Here's how the part is built. I have some questions about the finished solid (model axes, mm). A direction names the side the tool comes from. Give positions to 0.01 mm unless a question says otherwise; leave off trailing zeros. Loops run counter-clockwise (first coordinate to the right, second up) from the corner with the lowest first, then second, coordinate; pieces in that order, holes last. Notation, with made-up numbers: (-6.75, 2) - (44.25, 2) arc R19 cw to (44.25, 22) - close; hole circle Ø5 at (76, 9). An arc over 180 degrees is marked (long way). Use one line per item in the form item = value.
from build123d import *

# Parameters (mm, degrees)
SKETCH2_R           = 3.5
BOSS_EXTRUDE1_DEPTH = 8
SKETCH3_R           = 3.5
BOSS_EXTRUDE2_DEPTH = 18
SKETCH4_W           = 12.5
SKETCH4_H           = 8
SKETCH4_W_2         = 8.5
SKETCH4_H_2         = 4
BOSS_EXTRUDE3_DEPTH = 10
SKETCH5_W           = 12.5
SKETCH5_H           = 8
BOSS_EXTRUDE4_DEPTH = 1
FILLET2_R           = 2
SKETCH6_W           = 15.377134156
SKETCH6_H           = 9.300468084
CUT_EXTRUDE1_DEPTH  = 12


with BuildPart() as part:
    # Sketch2 → Boss-Extrude1 (new body)
    with BuildSketch(Plane.XY):
        Circle(SKETCH2_R)
        with BuildLine():
            Line((-1.237436867, -1.237436867), (1.237436867, -1.237436867))
            ThreePointArc((1.237436867, -1.237436867), (0, 1.75), (-1.237436867, -1.237436867))
        make_face(mode=Mode.SUBTRACT)
    extrude(amount=BOSS_EXTRUDE1_DEPTH)

    # Sketch3 → Boss-Extrude2 (add)
    with BuildSketch(Plane.XY.offset(8)):
        Circle(SKETCH3_R)
    extrude(amount=BOSS_EXTRUDE2_DEPTH)

    # Sketch4 → Boss-Extrude3 (add)
    with BuildSketch(Plane.XY.offset(26)):
        Rectangle(SKETCH4_W, SKETCH4_H)
        Rectangle(SKETCH4_W_2, SKETCH4_H_2, mode=Mode.SUBTRACT)
    extrude(amount=BOSS_EXTRUDE3_DEPTH)

    # Sketch5 → Boss-Extrude4 (add)
    with BuildSketch(Plane(origin=(0, 0, 26), x_dir=(-1, 0, 0), z_dir=(0, 0, -1))):
        Rectangle(SKETCH5_W, SKETCH5_H)
    extrude(amount=BOSS_EXTRUDE4_DEPTH)

    # Fillet2
    fillet2_edges = [part.edges().sort_by_distance(p)[0] for p in [
        (-6.25, -4, 30.5),
        (6.25, -4, 30.5),
        (6.25, 4, 30.5),
        (-6.25, 4, 30.5),
    ]]
    fillet(fillet2_edges, radius=FILLET2_R)

    # Sketch6 → Cut-Extrude1 (cut, through all)
    with BuildSketch(Plane(origin=(0, 0, 25), x_dir=(-1, 0, 0), z_dir=(0, 0, -1))):
        with Locations((-0.478823703, -0.270525698)):
            Rectangle(SKETCH6_W, SKETCH6_H)
    extrude(amount=-CUT_EXTRUDE1_DEPTH, mode=Mode.SUBTRACT)


solid = part.part
(1) For P1, Ø1.5, axis at x = -1, z = 5, coming from the +Y side, with a flat end and sliding along its axis, tell me the tip position at first contact or that it passes through.
Geometry says:
P1 = 3.49
(2) If we section it at C-C (z = 6.5): List the corners of the cut face in (x, y) for me.
Geometry says:
outline = circle Ø7 at (0, 0); hole (-1.24, -1.24) - (1.24, -1.24) arc R1.75 ccw (long way) to start
(3) If we section it at A-A (y = 0): List the corners of the cut face in (x, z) for me, plus the area to 3 significant figures.
Geometry says:
outline = (-3.5, 0) - (-1.75, 0) - (-1.75, 8) - (1.75, 8) - (1.75, 0) - (3.5, 0) - (3.5, 25) - (-3.5, 25) - close
area = 147 mm²
(4) If we section it at D-D (z = 19.75): List the corners of the cut face in (x, y) for me.
Geometry says:
outline = circle Ø7 at (0, 0)
(5) Thinking about a two-plate mould opening in Y: for faces 3 (the cylindrical face through (3.233, -1.341, 12.325)), 4 (the flat face through (0, -1.237, 4)), 5 (the flat face through (0, 0, 25)), which applies, pulls with the +Y half, pulls with the -Y half, needs draft (parallel to the pull), parting line crosses it, or undercut?
Geometry says:
face_3 = parting line crosses it
face_4 = undercut
face_5 = needs draft
(6) If we section it at B-B (x = 0): List the corners of the cut face in (y, z) for me.
Geometry says:
outline = (-3.5, 0) - (-1.24, 0) - (-1.24, 8) - (1.75, 8) - (1.75, 0) - (3.5, 0) - (3.5, 25) - (-3.5, 25) - close
(7) If I drill on probe 1 along X at (y, z) = (0, 3); probe 2 along Y at (x, z) = (0, 2.5); probe 3 along Z at (x, y) = (-1, 1.25), over which ranges is the centre line in solid material (lowest first)?
Geometry says:
probe_1 = -3.5 to -1.75, 1.75 to 3.5
probe_2 = -3.5 to -1.24, 1.75 to 3.5
probe_3 = 8 to 25
(8) For faces 1 (the cylindrical face through (0.06, 1.75, 3.94)), 2 (the flat face through (0, -2, 0)), which set-ups out of +Z, -Z, +X, -X, +Y, -Y let a thin tool reach every point of the face, with its end or its side?
Geometry says:
face_1 = -Z
face_2 = -Z, +X, -X, +Y, -Y
